Design review of the part built by this model. Coordinates are the model's own, in mm. Face numbers are marked on the shaded views. Coordinates: 2 decimals unless noted, no trailing zeros. Order: outer loops, then holes, each group sorted by start corner. A loop starts at its lowest first (then second) coordinate and runs counter-clockwise, first axis right, second up. Notation, with made-up numbers: M -34.75,-37 L 7.25,-37 A31 cw 7.25,-12 Z; hole C -2,81 d3. An arc over 180 degrees is marked long. Answer in a Markdown table with one row per item.
from build123d import *

# Parameters (mm, degrees)
SKETCH1_W           = 60
SKETCH1_H           = 114
BOSS_EXTRUDE1_DEPTH = 10
SKETCH3_W           = 60
SKETCH3_H           = 7
BOSS_EXTRUDE2_DEPTH = 111.6
BOSS_EXTRUDE5_DEPTH = 10
BOSS_EXTRUDE3_DEPTH = 10
SKETCH7_W           = 10
SKETCH7_H           = 7
CUT_EXTRUDE1_DEPTH  = 56.6
SKETCH8_R           = 3.175
CUT_EXTRUDE2_DEPTH  = 8


with BuildPart() as part:
    # Sketch1 → Boss-Extrude1 (new body)
    with BuildSketch(Plane(origin=(0, 0, 0), x_dir=(1, 0, 0), z_dir=(0, 1, 0))):
        Rectangle(SKETCH1_W, SKETCH1_H)
    extrude(amount=-BOSS_EXTRUDE1_DEPTH)

    # Sketch3 → Boss-Extrude2 (add)
    with BuildSketch(Plane(origin=(0, 0, 0), x_dir=(1, 0, 0), z_dir=(0, 1, 0))):
        with Locations((0, 53.5)):
            Rectangle(SKETCH3_W, SKETCH3_H)
    extrude(amount=BOSS_EXTRUDE2_DEPTH)

    # Sketch6 → Boss-Extrude5 (add)
    with BuildSketch(Plane(origin=(0, 0, 0), x_dir=(1, 0, 0), z_dir=(0, 1, 0))):
        Polygon((-30, 50), (-20, 50), (-20.103587149, -50), (30, -50), (30, -57), (-30, -57), align=None)
    extrude(amount=BOSS_EXTRUDE5_DEPTH)

    # Sketch4 → Boss-Extrude3 (add)
    with BuildSketch(Plane.ZY.offset(30)):
        Polygon((-57, 10), (57, 10), (-50, 111.6), (-57, 111.6), align=None)
    extrude(amount=-BOSS_EXTRUDE3_DEPTH)

    # Sketch7 → Cut-Extrude1 (cut)
    with BuildSketch(Plane(origin=(0, 111.6, 0), x_dir=(1, 0, 0), z_dir=(0, 1, 0))):
        with Locations((25, 53.5)):
            Rectangle(SKETCH7_W, SKETCH7_H)
    extrude(amount=-CUT_EXTRUDE1_DEPTH, mode=Mode.SUBTRACT)

    # Sketch8 → Cut-Extrude2 (cut, through all)
    with BuildSketch(Plane.XY.offset(-50)):
        with Locations((-10, 96.6)):
            Circle(SKETCH8_R)
        with Locations((7.3, 81.6)):
            Circle(SKETCH8_R)
        with Locations((-10, 66.6)):
            Circle(SKETCH8_R)
    extrude(amount=-CUT_EXTRUDE2_DEPTH, mode=Mode.SUBTRACT)


solid = part.part
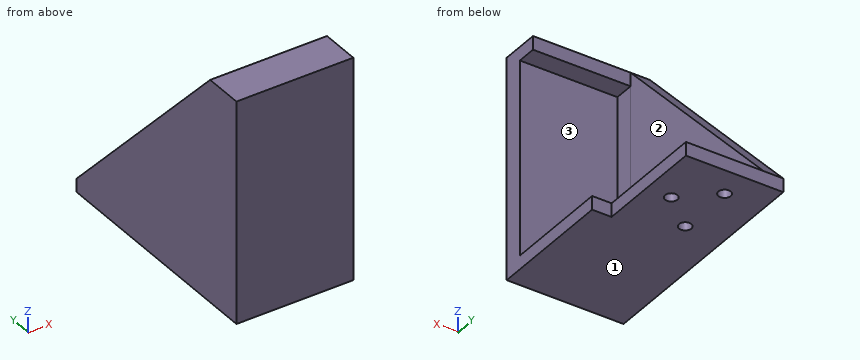
(1) Draft analysis for pull direction Z (two halves, no side actions). For the marked faces 1, 2 and 3, state which applies: pulls with the +Z half, pulls with the -Z half, needs draft (parallel to the pull), parting line crosses it, or undercut.
Return value:
| item | result |
|---|---|
| face 1 | pulls with the -Z half |
| face 2 | needs draft |
| face 3 | undercut |
(2) Insertion check: pin 1 Ø2 at (y, z) = (86, -40) entering from +X; pin 2 Ø8 at (x, z) = (8.5, 9) entering from +Y; pin 3 Ø3.5 at (y, z) = (83.5, -55) entering from +X. Each pin has a flat end and moves straight along its axis. Give the tip position at first contact, or say it passes through.
Return value:
| item | result |
|---|---|
| pin 1 | stops at x = -20 |
| pin 2 | stops at y = 0 |
| pin 3 | stops at x = 20 |
(3) For line 1 along Y through (x, z) = (-10, -55) (3 decimals); line 2 along Y through (x, z) = (7, -53); line 3 along Z through (x, y) = (-13, 4), list the stretches that pass through material, from the lowest coordinate up. Write a range as from..to.
Return value:
| item | result |
|---|---|
| line 1 | y = -10..63.425, 69.775..93.425, 99.775..111.6 |
| line 2 | y = -10..78.44, 84.76..111.6 |
| line 3 | z = -57..-50, 50..57 |
(4) Add section A-A, the plane x = 7.3. Give the boundary of the cut face in (y, z) (3 decimals), and give its area (3 significant figures).
Return value:
| item | result |
|---|---|
| outline | M -10,-57 L 78.425,-57 L 78.425,-50 L 0,-50 L 0,50 L 10,50 L 10,57 L -10,57 Z; M 84.775,-57 L 111.6,-57 L 111.6,-50 L 84.775,-50 Z |
| area | 1,950 mm2 |
(5) Add section B-B, the plane x = -10. Give the boundary of the cut face in (y, z) (3 decimals).
Return value:
| item | result |
|---|---|
| outline | M -10,-57 L 63.425,-57 L 63.425,-50 L 0,-50 L 0,50 L 10,50 L 10,57 L -10,57 Z; M 69.775,-57 L 93.425,-57 L 93.425,-50 L 69.775,-50 Z; M 99.775,-57 L 111.6,-57 L 111.6,-50 L 99.775,-50 Z |
(6) Add section C-C, the plane y = 66.6. Give the boundary of the cut face in (x, z) (3 decimals).
Return value:
| item | result |
|---|---|
| outline | M -30,-57 L -13.175,-57 L -13.175,-50 L -20,-50 L -20,-2.608 L -30,-2.608 Z; M -6.825,-57 L 20,-57 L 20,-50 L -6.825,-50 Z |
(7) Add section D-D, the plane z = 40. Give the boundary of the cut face in (x, y).
Return value:
| item | result |
|---|---|
| outline | M -30,-10 L 30,-10 L 30,0 L -20.09,0 L -20.09,10 L -20,10 L -20,26.14 L -30,26.14 Z |
